For this review, take the finished solid that the model builds, in its own axes (mm). A direction names the side the tool comes from. Round coordinates to 2 decimals unless told otherwise and drop trailing zeros. Write each loop counter-clockwise with the first axis right and the second up, starting at its lowest first coordinate (ties: lowest second). Pieces come first, ordered by that corner, then holes. Notation, with made-up numbers: (58.25, 64) -> (97.25, 64) arc R32 cw to (97.25, 99) -> close; hole circle Ø8 at (-26, 63). An arc over 180 degrees is marked (long way). Answer in a Markdown table with one row per item. Add a question column.
```python
from build123d import *

# Parameters (mm, degrees)
ESQUISSE1_W             = 300
ESQUISSE1_H             = 60
BOSS_EXTRU_1_DEPTH      = 8
ESQUISSE2_W             = 15.862965147
ESQUISSE2_H             = 8
ESQUISSE2_W_2           = 15
ENL_V_MAT_EXTRU_1_DEPTH = 8


with BuildPart() as part:
    # Esquisse1 → Boss.-Extru.1 (new body)
    with BuildSketch(Plane.XY):
        Rectangle(ESQUISSE1_W, ESQUISSE1_H)
    extrude(amount=BOSS_EXTRU_1_DEPTH)

    # Esquisse2 → Enlèv. mat.-Extru.1 (cut)
    with BuildSketch(Plane.XY):
        Polygon((-0.862965147, -30), (15, -30), (15, -22), (-0.862965147, -22), (-15.862965147, -22), (-15.862965147, -30), align=None)
        with Locations((37.068517427, -26)):
            Rectangle(ESQUISSE2_W, ESQUISSE2_H)
        with Locations((67.068517426, -26)):
            Rectangle(ESQUISSE2_W, ESQUISSE2_H)
        with Locations((97.068517426, -26)):
            Rectangle(ESQUISSE2_W, ESQUISSE2_H)
        with Locations((127.068517426, -26)):
            Rectangle(ESQUISSE2_W, ESQUISSE2_H)
        with Locations((-127.5, -26)):
            Rectangle(ESQUISSE2_W_2, ESQUISSE2_H)
        with Locations((-97.5, -26)):
            Rectangle(ESQUISSE2_W_2, ESQUISSE2_H)
        with Locations((-67.5, -26)):
            Rectangle(ESQUISSE2_W_2, ESQUISSE2_H)
        with Locations((-37.5, -26)):
            Rectangle(ESQUISSE2_W_2, ESQUISSE2_H)
    extrude(amount=ENL_V_MAT_EXTRU_1_DEPTH, mode=Mode.SUBTRACT)


solid = part.part
```
1. Clearance check with a flat-ended pin moving along its axis: pin 1 Ø2.5 at (x, z) = (34.5, 4) entering from -Y. State where the tip first meets the part, or that it passes through.
2. For L1, parallel to Y at x = 38.5, z = 3.5, list the stretches that pass through material, from the lowest coordinate up. Write a range as [from, to].
3. The part is to be moulded in two halves that separate along X. For faces 1 (the flat face through (-2, 0, 8)), 2 (the flat face through (75, -26, 4)), 3 (the flat face through (-60, -26, 4)), say which applies: pulls with the +X half, pulls with the -X half, needs draft (parallel to the pull), parting line crosses it, or undercut.
4. Tool access review of faces 4 (the flat face through (22, -30, 4)), 5 (the flat face through (-30, -26, 4)): name each direction out of +Z, -Z, +X, -X, +Y, -Y from which nothing blocks a thin tool from reaching the whole face with its end or side.
5. We need section A-A (x = 124.5). Write out the cut boundary in (y, z), plus the area to 3 significant figures.
Response:
| question | item | result |
|---|---|---|
| 1 | pin 1 | y = -22 |
| 2 | L1 | [-22, 30] |
| 3 | face 1 | needs draft |
| 3 | face 2 | undercut |
| 3 | face 3 | undercut |
| 4 | face 4 | +Z, -Z, +X, -X, -Y |
| 4 | face 5 | +Z, -Z, -Y |
| 5 | outline | (-22, 0) -> (30, 0) -> (30, 8) -> (-22, 8) -> close |
| 5 | area | 416 mm2 |
